Source: three-view drawing plus pictorial views. Frame: mm from the lowest corner of the part. Round coordinates to 2 decimals unless told otherwise and drop trailing zeros. Loops run counter-clockwise (first coordinate to the right, second up) from the corner with the lowest first, then second, coordinate; pieces in that order, holes last. Notation, with made-up numbers: M -24.75,83.25 L 27.25,83.25 A29 cw 27.25,103.25 Z; hole C 5,-7.5 d10. An arc over 180 degrees is marked long. Answer as a JSON object with one key per item and string values.
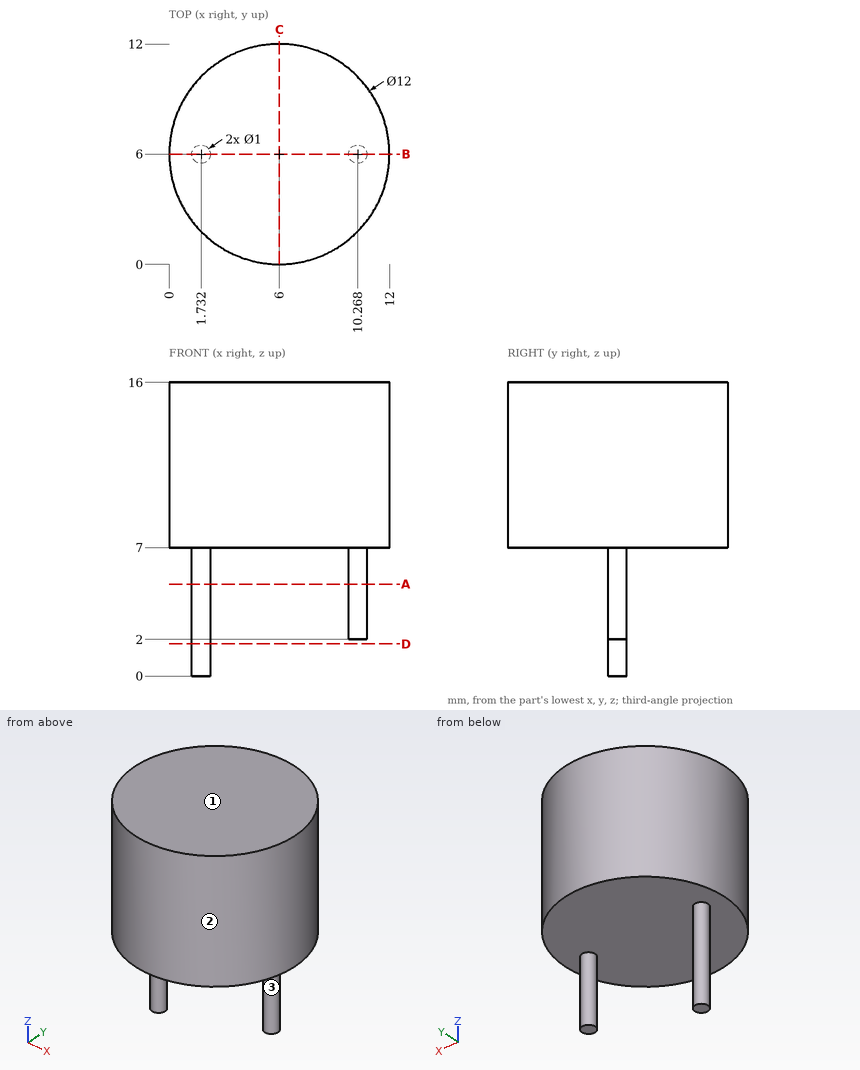
1) First-contact query: pin 1 (4 mm diameter, centred on x = 10, z = 2, fed in from +Y); pin 2 (0.8 mm diameter, centred on x = 10, y = 6, fed in from -Z). Flat tips, straight axial feed; report the tip coordinate or a pass-through.
Geometry results:
{"pin 1": "y = 6.5", "pin 2": "z = 2"}
2) Line query: probe 1 along Z at (x, y) = (9.25, 3.75); probe 2 along X at (y, z) = (6.25, 4.5) (1 decimal); probe 3 along Y at (x, z) = (1, 9.25) (1 decimal). Output: solid intervals per line, ascending.
Geometry results:
{"probe 1": "7 to 16", "probe 2": "1.3 to 2.2, 9.8 to 10.7", "probe 3": "2.7 to 9.3"}
3) Cut plane A-A on z = 5. Return the cut outline in (x, y), and give its area (3 significant figures).
Geometry results:
{"outline": "C 1.73,6 d1; C 10.27,6 d1", "area": "1.57 mm2"}
4) Cut plane D-D on z = 1.75. Return the cut outline in (x, y).
Geometry results:
{"outline": "C 1.73,6 d1"}
5) Cut plane C-C on x = 6. Return the cut outline in (y, z).
Geometry results:
{"outline": "M 0,7 L 12,7 L 12,16 L 0,16 Z"}
6) Cut plane B-B on y = 6. Return the cut outline in (x, z).
Geometry results:
{"outline": "M 0,7 L 1.23,7 L 1.23,0 L 2.23,0 L 2.23,7 L 9.77,7 L 9.77,2 L 10.77,2 L 10.77,7 L 12,7 L 12,16 L 0,16 Z"}
7) Pull-direction query (X, two-part tool) for the marked faces 1, 2 and 3; classes: +X half, -X half, draft (parallel to the pull), parting line (faces both ways), or undercut.
Geometry results:
{"face 1": "draft", "face 2": "parting line", "face 3": "undercut"}
